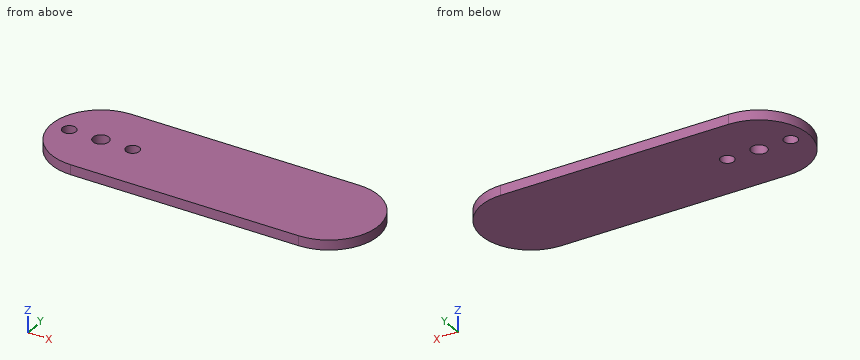
from build123d import *

# Parameters (mm, degrees)
SKETCH2_R           = 4
SKETCH2_R_2         = 3.4
BOSS_EXTRUDE1_DEPTH = 2.5


with BuildPart() as part:
    # Sketch2 → Boss-Extrude1 (new, symmetric)
    with BuildSketch(Plane.XY):
        with BuildLine():
            Line((0, 25), (115, 25))
            ThreePointArc((115, 25), (140, 0), (115, -25))
            Line((115, -25), (0, -25))
            ThreePointArc((0, -25), (-25, 0), (0, 25))
        make_face()
        Circle(SKETCH2_R, mode=Mode.SUBTRACT)
        with Locations((16, 0)):
            Circle(SKETCH2_R_2, mode=Mode.SUBTRACT)
        with Locations((-16, 0)):
            Circle(SKETCH2_R_2, mode=Mode.SUBTRACT)
    extrude(amount=BOSS_EXTRUDE1_DEPTH, both=True)


solid = part.part
Work out the finished part from the listing and answer in its coordinate system (mm). Coordinates: 2 decimals unless noted, no trailing zeros. Write each loop counter-clockwise with the first axis right and the second up, starting at its lowest first coordinate (ties: lowest second). Pieces come first, ordered by that corner, then holes. Notation, with made-up numbers: M 83.5,73.25 L 111.5,73.25 A28 ccw 111.5,102.25 Z; hole C 55.25,5.25 d8. An arc over 180 degrees is marked long. Write item = value, one per line.
1. Straight lines are drawn through the part: line 1 (Y direction, x = 0, z = -0.2); line 2 (Y direction, x = 16, z = -1.15); line 3 (Y direction, x = -12, z = 2). For each, find the intervals that lie inside material, in ascending order. Write a range as from..to.
Solution:
line_1 = -25..-4, 4..25
line_2 = -25..-3.4, 3.4..25
line_3 = -21.93..21.93
2. Flat-ended cylindrical pins translate along their axes: pin 1 (10.5 mm diameter, centred on x = 0, y = 0, fed in from -Z); pin 2 (2 mm diameter, centred on y = 19, z = 1.5, fed in from +X); pin 3 (4 mm diameter, centred on x = 16, y = 0, fed in from +Z); pin 4 (2 mm diameter, centred on y = -14, z = -1.5, fed in from +X). Find the tip coordinate at first contact, or state that the pin passes through.
Solution:
pin_1 = -2.5
pin_2 = 132.35
pin_3 = through
pin_4 = 136.35
3. The part is cut by section D-D (x = -16). Determine the outline of the cut face in (y, z).
Solution:
outline = M -19.21,-2.5 L -3.4,-2.5 L -3.4,2.5 L -19.21,2.5 Z; M 3.4,-2.5 L 19.21,-2.5 L 19.21,2.5 L 3.4,2.5 Z
4. The part is cut by section A-A (y = 0). Determine the outline of the cut face in (x, z).
Solution:
outline = M -25,-2.5 L -19.4,-2.5 L -19.4,2.5 L -25,2.5 Z; M -12.6,-2.5 L -4,-2.5 L -4,2.5 L -12.6,2.5 Z; M 4,-2.5 L 12.6,-2.5 L 12.6,2.5 L 4,2.5 Z; M 19.4,-2.5 L 140,-2.5 L 140,2.5 L 19.4,2.5 Z
5. The part is cut by section C-C (x = 16). Determine the outline of the cut face in (y, z).
Solution:
outline = M -25,-2.5 L -3.4,-2.5 L -3.4,2.5 L -25,2.5 Z; M 3.4,-2.5 L 25,-2.5 L 25,2.5 L 3.4,2.5 Z
6. The part is cut by section B-B (z = 0.05). Determine the outline of the cut face in (x, y), then the cut area to 3 significant figures.
Solution:
outline = M 0,-25 L 115,-25 A25 ccw 115,25 L 0,25 A25 ccw Z; hole C -16,0 d6.8; hole C 0,0 d8; hole C 16,0 d6.8
area = 7,590 mm2
